Solid Edge part; units mm, degrees
sketch "Sketch1" plane through (0, 0, 0) normal (0, -1, 0) x (1, 0, 0)
  line L0 (4.0474, 0.14) -> (1.9025, 3.5751)
  line L1 (1.9025, 3.5751) -> (-2.1449, 3.4351)
  line L2 (-2.1449, 3.4351) -> (-4.0474, -0.14)
  line L3 (-4.0474, -0.14) -> (-1.9025, -3.5751)
  line L4 (-1.9025, -3.5751) -> (2.1449, -3.4351)
  line L5 (2.1449, -3.4351) -> (4.0474, 0.14)
extrude "Protrusion1" add sketch "Sketch1" against normal blind 2.5
sketch "Sketch2" plane through (0, 2.5, 0) normal (0, 1, 0) x (0.4698, 0, 0.8828)
  circle A0 centre (0, 0) radius 5
extrude "ExtrudedProtrusion_4" add sketch "Sketch2" along normal blind 0.5
sketch "Sketch3" plane through (0, 2.5, 0) normal (0, 1, 0) x (0.4698, 0, 0.8828)
  circle A0 centre (0, 0) radius 2.5
extrude "ExtrudedProtrusion_5" add sketch "Sketch3" along normal blind 10
sketch "Sketch4" plane through (1.5498, 1.5498, 0) normal (0, 0, -1) x (-1, 0, 0)
  line L0 (-1.9502, -1.562) -> (-3.6822, -0.562)
  line L1 (1.5498, -1.562) -> (-1.9502, -1.562)
  line L2 (1.5498, -1.562) -> (1.5498, -1.5498)
revolve "RevolvedCutout1" cut sketch "Sketch4" angle 360 about axis through (0, -3.0266, 0) along (0, 1, 0) material side at (4.391, 0.4445, 0)
Part model, mm, in its own coordinate system. A direction names the side the tool comes from. Round coordinates to 2 decimals unless told otherwise and drop trailing zeros. Loops run counter-clockwise (first coordinate to the right, second up) from the corner with the lowest first, then second, coordinate; pieces in that order, holes last.
1. Flat gauge pins, fed straight in: pin 1 (1.5 mm diameter, centred on x = -3, y = 2.5, fed in from +Z); pin 2 (6 mm diameter, centred on x = -3.5, y = 10, fed in from +Z); pin 3 (6 mm diameter, centred on x = -1.5, y = 5.5, fed in from -Z); pin 4 (2 mm diameter, centred on x = -0.5, z = 3.5, fed in from +Y). Where does each tip first touch, or does it go through?
Solutions:
pin 1: stops at z = 4.47
pin 2: stops at z = 2.45
pin 3: stops at z = -5
pin 4: stops at y = 3
2. Slice it at D-D (z = -1.75). Give the cut face in (x, y).
Solutions:
outline: (-4.68, 2.5) - (-3.04, 2.5) - (-3.04, 0) - (3.04, 0) - (3.04, 2.5) - (4.68, 2.5) - (4.68, 3) - (1.79, 3) - (1.79, 12.5) - (-1.79, 12.5) - (-1.79, 3) - (-4.68, 3) - close
3. Slice it at A-A (y = 1.25). Give the cut face in (x, z).
Solutions:
outline: (-4.05, -0.14) - (-1.9, -3.58) - (2.14, -3.44) - (4.05, 0.14) - (1.9, 3.58) - (-2.14, 3.44) - close
4. Drill centre lines: line 1 along Y through (x, z) = (1.25, -3.25); line 2 along Y through (x, z) = (4.75, 0.75); line 3 along Z through (x, y) = (1, 8.25). Where is each one in solid material? Low to high.
Solutions:
line 1: y = 0 to 3
line 2: y = 2.5 to 3
line 3: z = -2.29 to 2.29
5. 3-axis set-ups, long thin cutter, end or side, ignore diameter. For faces 1 (the face through (-3.083, 1.232, 1.673)), 2 (the face through (-2.99, 1.23, -1.83)), 3 (the face through (-2, 3, 2)): which of +Z, -Z, +X, -X, +Y, -Y reach the whole face in a straight line?
Solutions:
face 1: +Z, -X, -Y
face 2: -Z, -X, -Y
face 3: +Y
6. Slice it at B-B (z = -4). Give the cut face in (x, y).
Solutions:
outline: (-3, 2.5) - (3, 2.5) - (3, 3) - (-3, 3) - close
7. Slice it at C-C (x = 0). Give the cut face in (y, z), and give its area (3 significant figures).
Solutions:
outline: (0, -3.51) - (2.5, -3.51) - (2.5, -5) - (3, -5) - (3, -2.5) - (12.5, -2.5) - (12.5, 2.5) - (3, 2.5) - (3, 5) - (2.5, 5) - (2.5, 3.51) - (0, 3.51) - close
area: 70.0 mm2
